Check sheet for the modelled part. Datum: model origin and axes. Units: mm. Give positions to 0.01 mm unless a question says otherwise; leave off trailing zeros. Order: outer loops, then holes, each group sorted by start corner. A loop starts at its lowest first (then second) coordinate and runs counter-clockwise, first axis right, second up. Notation, with made-up numbers: M 68,-24.75 L 123,-24.75 A23 cw 123,-10.75 Z; hole C 9,17 d8. An arc over 180 degrees is marked long. Answer in a Markdown table with one row per item. Add a question column.
from build123d import *

# Parameters (mm, degrees)
SKETCH_1_W          = 121.4
SKETCH_1_H          = 128.7
EXTRUDE_1_DEPTH     = 1.5
EXTRUDE_2_DEPTH     = 2
SKETCH_3_W          = 1.5
SKETCH_3_H          = 96.8
SKETCH_3_W_2        = 113.8
SKETCH_3_H_2        = 1.5
EXTRUDE_3_DEPTH     = 2
SKETCH_5_W          = 121.4
SKETCH_5_H          = 8
SKETCH_5_W_2        = 12.45
SKETCH_5_H_2        = 4.8
SKETCH_5_W_3        = 9.05
SKETCH_5_W_4        = 17.75
SKETCH_5_W_5        = 14.35
SKETCH_5_W_6        = 48
EXTRUDE_5_DEPTH     = 4
SKETCH_7_R          = 4.75
EXTRUDE_10_DEPTH    = 4
SKETCH_8_R          = 1.75
CUT_EXTRUDE_3_DEPTH = 5.5
CHAMFER_1_SIZE      = 1.6
SKETCH_10_W         = 48
SKETCH_10_H         = 6.5
CUT_EXTRUDE_4_DEPTH = 4
CHAMFER_2_SIZE      = 0.5
CHAMFER_2_SIZE2     = 0.866025404


with BuildPart() as part:
    # Эскиз1 → Бобышка-Вытянуть1 (new body)
    with BuildSketch(Plane(origin=(0, 0, 0), x_dir=(1, 0, 0), z_dir=(0, 1, 0))):
        with Locations((60.7, 64.35)):
            Rectangle(SKETCH_1_W, SKETCH_1_H)
    extrude(amount=EXTRUDE_1_DEPTH)

    # Эскиз2 → Бобышка-Вытянуть2 (add)
    with BuildSketch(Plane(origin=(0, 1.5, 0), x_dir=(1, 0, 0), z_dir=(0, 1, 0))):
        Polygon((0, 8), (0, 128.7), (121.4, 128.7), (121.4, 8), (117.6, 8), (117.6, 124.9), (3.8, 124.9), (3.8, 8), align=None)
    extrude(amount=EXTRUDE_2_DEPTH)

    # Эскиз3 → Бобышка-Вытянуть3 (add)
    with BuildSketch(Plane(origin=(0, 3.5, 0), x_dir=(1, 0, 0), z_dir=(0, 1, 0))):
        Polygon((0, 8), (3.8, 8), (3.8, 124.9), (117.6, 124.9), (117.6, 8), (121.4, 8), (121.4, 128.7), (0, 128.7), align=None)
        with Locations((1.85, 59)):
            Rectangle(SKETCH_3_W, SKETCH_3_H, mode=Mode.SUBTRACT)
        with Locations((60.7, 126.85)):
            Rectangle(SKETCH_3_W_2, SKETCH_3_H_2, mode=Mode.SUBTRACT)
        with Locations((119.55, 59)):
            Rectangle(SKETCH_3_W, SKETCH_3_H, mode=Mode.SUBTRACT)
    extrude(amount=EXTRUDE_3_DEPTH)

    # Эскиз5 → Бобышка-Вытянуть5 (add)
    with BuildSketch(Plane(origin=(0, 1.5, 0), x_dir=(1, 0, 0), z_dir=(0, 1, 0))):
        with Locations((60.7, 4)):
            Rectangle(SKETCH_5_W, SKETCH_5_H)
        with Locations((7.925, 3.9)):
            Rectangle(SKETCH_5_W_2, SKETCH_5_H_2, mode=Mode.SUBTRACT)
        with Locations((115.175, 3.9)):
            Rectangle(SKETCH_5_W_3, SKETCH_5_H_2, mode=Mode.SUBTRACT)
        with Locations((95.275, 3.9)):
            Rectangle(SKETCH_5_W_4, SKETCH_5_H_2, mode=Mode.SUBTRACT)
        with Locations((27.825, 3.9)):
            Rectangle(SKETCH_5_W_5, SKETCH_5_H_2, mode=Mode.SUBTRACT)
        with Locations((60.7, 3.9)):
            Rectangle(SKETCH_5_W_6, SKETCH_5_H_2, mode=Mode.SUBTRACT)
    extrude(amount=EXTRUDE_5_DEPTH)

    # Эскиз7 → Бобышка-Вытянуть10 (add)
    with BuildSketch(Plane(origin=(0, 1.5, 0), x_dir=(1, 0, 0), z_dir=(0, 1, 0))):
        with Locations((5.95, 115)):
            Circle(SKETCH_7_R)
        with Locations((115.45, 115)):
            Circle(SKETCH_7_R)
        with Locations((15.2, 4.75)):
            Circle(SKETCH_7_R)
        with Locations((106.2, 4.75)):
            Circle(SKETCH_7_R)
    extrude(amount=EXTRUDE_10_DEPTH)

    # Эскиз8 → Вырез-Вытянуть3 (cut)
    with BuildSketch(Plane.XZ):
        with Locations(Location((15.2, -4.75, 0), (0, 0, 270))):
            Circle(SKETCH_8_R)
        with Locations(Location((106.2, -4.75, 0), (0, 0, 270))):
            Circle(SKETCH_8_R)
        with Locations(Location((5.95, -115, 0), (0, 0, 270))):
            Circle(SKETCH_8_R)
        with Locations(Location((115.45, -115, 0), (0, 0, 270))):
            Circle(SKETCH_8_R)
    extrude(amount=-CUT_EXTRUDE_3_DEPTH, mode=Mode.SUBTRACT)

    # Фаска1
    chamfer_1_edges = [part.edges().sort_by_distance(p)[0] for p in [
        (115.45, 0, -113.25),
        (5.95, 0, -113.25),
        (106.2, 0, -3),
        (15.2, 0, -3),
    ]]
    chamfer(chamfer_1_edges, length=CHAMFER_1_SIZE)

    # Эскиз10 → Вырез-Вытянуть4 (cut)
    with BuildSketch(Plane(origin=(0, 5.5, 0), x_dir=(1, 0, 0), z_dir=(0, 1, 0))):
        with Locations((60.7, 4.75)):
            Rectangle(SKETCH_10_W, SKETCH_10_H)
    extrude(amount=-CUT_EXTRUDE_4_DEPTH, mode=Mode.SUBTRACT)

    # Фаска2
    chamfer_2_edges = [part.edges().sort_by_distance(p)[0] for p in [
        (0, 0, -64.35),
        (60.7, 0, -128.7),
        (121.4, 0, -64.35),
        (60.7, 0, 0),
    ]]
    chamfer_2_side = [part.faces().sort_by_distance(p)[0] for p in [
        (60.7, 0, -64.390759898),
    ]]
    chamfer(chamfer_2_edges, length=CHAMFER_2_SIZE, length2=CHAMFER_2_SIZE2, reference=chamfer_2_side[0])


solid = part.part
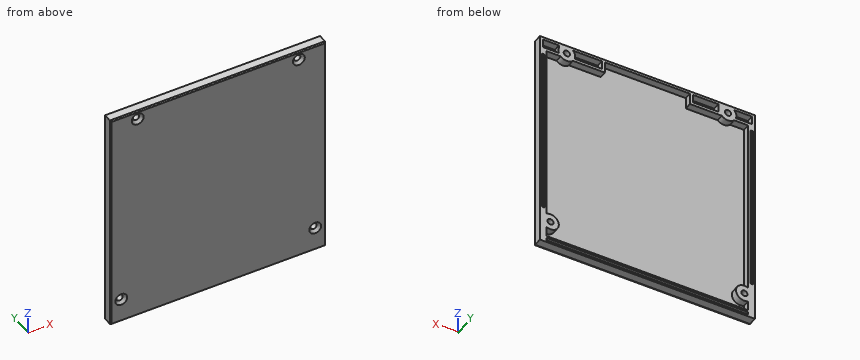
Q1. Thickness scan on probe 1 along Z at (x, y) = (106.2, 3.75); probe 2 along Z at (x, y) = (95, 4.95); probe 3 along Z at (x, y) = (115.45, 4.1). Record the ranges inside material, lowest first.
Q2. Go/stop test with a flat-tipped pin: pin 1 (2.5 mm diameter, centred on x = 31, z = -4.5, fed in from +Y). Record where the tip stops, or that it passes through.
Q3. Cross-section at B-B (x = 5.95). Record the boundary of the cut face in (y, z).
Q4. Cross-section at C-C (x = 40.5). Record the boundary of the cut face in (y, z), and give its area (3 significant figures).
Q5. Cross-section at D-D (z = -48). Record the boundary of the cut face in (x, y), and give its area (3 significant figures).
Q6. Cross-section at A-A (z = -115). Record the boundary of the cut face in (x, y), and give its area (3 significant figures).
Values follow:
| question | item | result |
|---|---|---|
| 1 | probe 1 | -128.7 to -127.6, -126.1 to -124.9, -9.5 to -6.5, -3 to 0 |
| 1 | probe 2 | -128.7 to -127.6, -126.1 to -124.9, -8 to -6.3, -1.5 to 0 |
| 1 | probe 3 | -128.7 to -127.6, -126.1 to -124.9, -119.75 to -116.75, -113.25 to -110.25, -8 to -6.3, -1.5 to 0 |
| 2 | pin 1 | y = 1.5 |
| 3 | outline | M 0,-128.2 L 0.87,-128.7 L 5.5,-128.7 L 5.5,-127.6 L 3.5,-127.6 L 3.5,-126.1 L 5.5,-126.1 L 5.5,-124.9 L 1.5,-124.9 L 1.5,-119.75 L 5.5,-119.75 L 5.5,-116.75 L 1.6,-116.75 L 0,-118.35 Z; M 0,-111.65 L 1.6,-113.25 L 5.5,-113.25 L 5.5,-110.25 L 1.5,-110.25 L 1.5,-8 L 5.5,-8 L 5.5,-6.3 L 1.5,-6.3 L 1.5,-1.5 L 5.5,-1.5 L 5.5,0 L 0.87,0 L 0,-0.5 Z |
| 4 | outline | M 0,-128.2 L 0.87,-128.7 L 5.5,-128.7 L 5.5,-127.6 L 3.5,-127.6 L 3.5,-126.1 L 5.5,-126.1 L 5.5,-124.9 L 1.5,-124.9 L 1.5,-1.5 L 5.5,-1.5 L 5.5,0 L 0.87,0 L 0,-0.5 Z |
| 4 | area | 211 mm² |
| 5 | outline | M 0,0.87 L 0.5,0 L 120.9,0 L 121.4,0.87 L 121.4,5.5 L 120.3,5.5 L 120.3,3.5 L 118.8,3.5 L 118.8,5.5 L 117.6,5.5 L 117.6,1.5 L 3.8,1.5 L 3.8,5.5 L 2.6,5.5 L 2.6,3.5 L 1.1,3.5 L 1.1,5.5 L 0,5.5 Z |
| 5 | area | 206 mm² |
| 6 | outline | M 0,0.87 L 0.5,0 L 2.6,0 L 4.2,1.6 L 4.2,5.5 L 0,5.5 Z; M 7.7,1.6 L 9.3,0 L 112.1,0 L 113.7,1.6 L 113.7,5.5 L 110.7,5.5 L 110.7,1.5 L 10.7,1.5 L 10.7,5.5 L 7.7,5.5 Z; M 117.2,1.6 L 118.8,0 L 120.9,0 L 121.4,0.87 L 121.4,5.5 L 117.2,5.5 Z |
| 6 | area | 224 mm² |
